The drawing under review shows one solid part. Ordinate dimensions are in mm from its lowest x, y, z. A direction names the side the tool comes from. Coordinates: 2 decimals unless noted, no trailing zeros. Write each loop counter-clockwise with the first axis right and the second up, starting at its lowest first coordinate (ties: lowest second). Pieces come first, ordered by that corner, then holes. Notation, with made-up numbers: M 73.25,2 L 80.25,2 A30 ccw 80.25,25 Z; hole C 5,14.25 d4. An arc over 180 degrees is marked long. Answer as CSV lines item,"result". Start each with the question number.
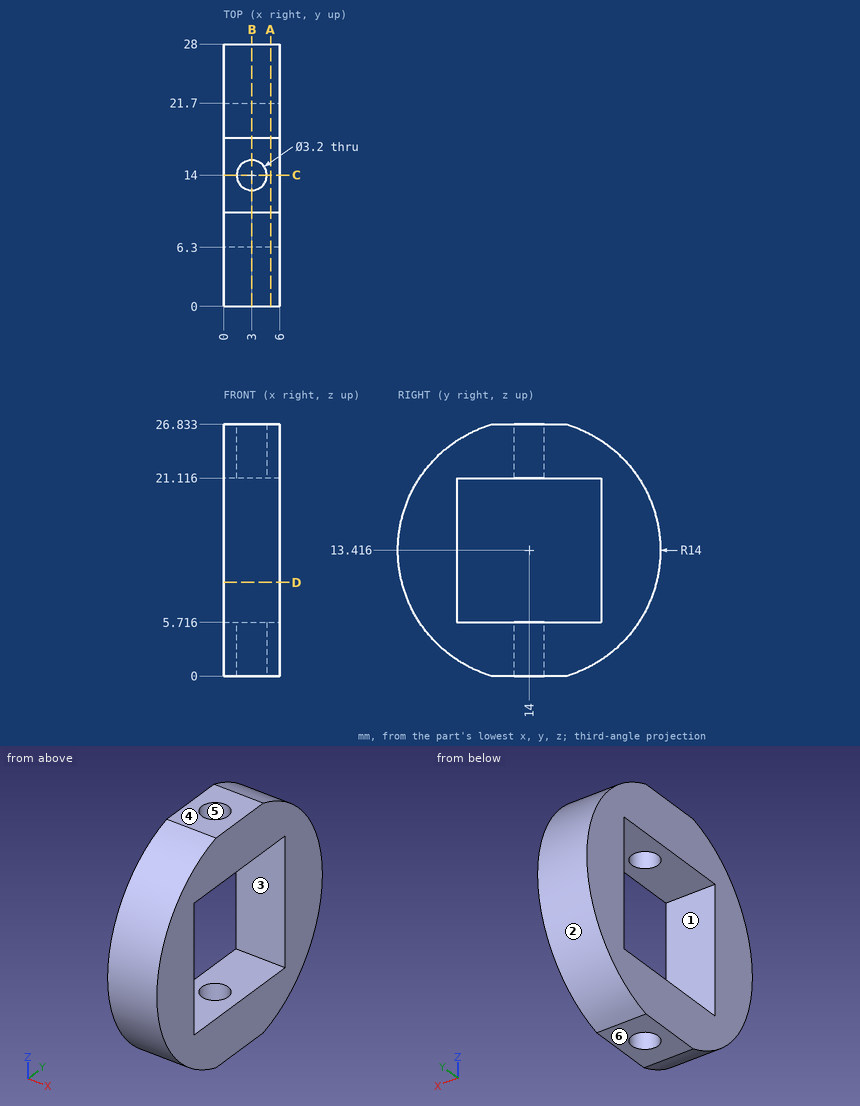
1) Mouldability with a two-part tool opening along Z and no side actions: class the marked faces 3, 4, 5 and 6 as +Z half, -Z half, draft (parallel to the pull), parting line (faces both ways), or undercut.
2) Take a section at D-D on z = 10. Give the boundary of the cut face in (x, y).
3) Take a section at A-A on x = 5. Give the boundary of the cut face in (y, z).
4) Take a section at C-C on y = 14. Give the boundary of the cut face in (x, z).
5) Tool access review of the marked faces 1 and 2: name each direction out of +Z, -Z, +X, -X, +Y, -Y from which nothing blocks a thin tool from reaching the whole face with its end or side.
6) Clearance check with flat-ended pins moving along their axes: pin 1 Ø1 at (x, z) = (0.5, 15.5) entering from -Y; pin 2 Ø1.9 at (x, y) = (3, 14) entering from -Z; pin 3 Ø1.5 at (x, y) = (3.5, 22) entering from -Z. State where each tip first meets the part, or that it passes through.
7) Take a section at B-B on x = 3. Give the boundary of the cut face in (y, z), and give its area (3 significant figures).
8) To check wall thickness, follow line 1 (Z direction, x = 4.7, y = 16.75); line 2 (Y direction, x = 5.5, z = 18.5) (1 decimal); line 3 (Y direction, x = 3.55, z = 13.25). State the ranges of each line that lie inside material, in increasing order. Write a range as [from, to].
Results:
1,face 3,"undercut"
1,face 4,"+Z half"
1,face 5,"draft"
1,face 6,"-Z half"
2,outline,"M 0,0.42 L 6,0.42 L 6,6.3 L 0,6.3 Z; M 0,21.7 L 6,21.7 L 6,27.58 L 0,27.58 Z"
3,outline,"M 10,0 L 18,0 A14 ccw 18,26.83 L 10,26.83 A14 ccw Z; hole M 6.3,5.72 L 21.7,5.72 L 21.7,21.12 L 6.3,21.12 Z"
4,outline,"M 0,0 L 1.4,0 L 1.4,5.72 L 0,5.72 Z; M 0,21.12 L 1.4,21.12 L 1.4,26.83 L 0,26.83 Z; M 4.6,0 L 6,0 L 6,5.72 L 4.6,5.72 Z; M 4.6,21.12 L 6,21.12 L 6,26.83 L 4.6,26.83 Z"
5,face 1,"+X, -X"
5,face 2,"+X, -X, +Y"
6,pin 1,"stops at y = 0.09"
6,pin 2,"passes through"
6,pin 3,"stops at z = 1.44"
7,outline,"M 6.3,5.72 L 6.3,21.12 L 12.4,21.12 L 12.4,26.83 L 10,26.83 A14 ccw 10,0 L 12.4,0 L 12.4,5.72 Z; M 15.6,0 L 18,0 A14 ccw 18,26.83 L 15.6,26.83 L 15.6,21.12 L 21.7,21.12 L 21.7,5.72 L 15.6,5.72 Z"
7,area,"336 mm²"
8,line 1,"z = [0, 5.72], [21.12, 26.83]"
8,line 2,"y = [1, 6.3], [21.7, 27]"
8,line 3,"y = [0, 6.3], [21.7, 28]"
